Here's how the part is built. I have some questions about the finished solid (model axes, mm). A direction names the side the tool comes from. Give positions to 0.01 mm unless a question says otherwise; leave off trailing zeros. Write each loop counter-clockwise with the first axis right and the second up, starting at its lowest first coordinate (ties: lowest second). Pieces come first, ordered by that corner, then holes. Notation, with made-up numbers: M 55.5,25.5 L 77.5,25.5 A19 cw 77.5,56.5 Z; hole C 27,-11.75 d7. An arc over 180 degrees is marked long. Use one line per item in the form item = value. Start each with the question number.
from build123d import *

# Parameters (mm, degrees)
F1_DEPTH   = 228.6
F2_T       = -2.54
F4_W       = 223.52
F4_H       = 121.926114556
F5_DEPTH   = 134.112
F7_W       = 76.2
F7_H       = 177.8
F9_W       = 76.2
F9_H       = 177.8
F10_DEPTH  = 381
F8_FACE1_W = 76.2
F8_FACE1_H = 103.6678810409
F13_T      = -2.54
F11_W      = 533.4
F11_H      = 304.8
F11_W_2    = 76.2
F11_H_2    = 177.8
F14_DEPTH  = 5.08


# Not quite as in the source:
# - a shell that OpenCascade refuses in one call is made with other operations: the cavity is built on its own and cut out
# - a feature names something its author has since deleted; it is built from what else it names


with BuildPart() as f1:
    # F0 (on Right) → F1 (new body)
    with BuildSketch(Plane.YZ):
        Polygon((-381, 683.26), (0, 0), (145.4103401064, 0), (-235.5896598936, 683.26), align=None)
    extrude(amount=F1_DEPTH)

    # F2
    f2_openings = [f1.faces().sort_by_distance(p)[0] for p in [
        (114.3, -308.29483, 683.26),
    ]]
    offset(amount=F2_T, openings=f2_openings)

    # F4 (on face) → F5 (cut)
    with BuildSketch(Plane(origin=(0, 34.4790739886, -61.8450267372), x_dir=(1, 0, 0), z_dir=(0, -0.4869452699, 0.873432484))):
        with Locations((114.3, 63.503057278)):
            Rectangle(F4_W, F4_H)
    extrude(amount=F5_DEPTH, mode=Mode.SUBTRACT)

    # F7 (on offset) → F8 (join, up to the next surface of F1)
    with BuildSketch(Plane.XZ.offset(231.14)):
        with Locations((114.3, 139.7)):
            Rectangle(F7_W, F7_H)
    extrude(until=Until.NEXT, dir=(0, 1, 0))

    # F9 (on face) → F10 (join)
    with BuildSketch(Plane(origin=(0, 0, 50.8), x_dir=(1, 0, 0), z_dir=(0, 0, -1))):
        with Locations((114.3, 142.24)):
            Rectangle(F9_W, F9_H)
    extrude(amount=F10_DEPTH)

    # F8_face1 (on face) → F12 (join, up to the next surface of F1)
    with BuildSketch(Plane(origin=(114.3, -179.3060594796, 228.6), x_dir=(1, 0, 0), z_dir=(0, 0, 1))):
        Rectangle(F8_FACE1_W, F8_FACE1_H)
    extrude(until=Until.NEXT)

    # F13: a shell. OpenCascade refuses it in one call, so the cavity is built on its own and cut out:
    # the body offset inwards by the wall thickness, plus a prism from it out through each open face.
    f13_core = offset(f1.part, amount=F13_T, kind=Kind.INTERSECTION, mode=Mode.PRIVATE)
    f13_exits = [f13_core.faces().sort_by_distance(p)[0] for p in [
        (114.3, -55.88, -137.16),
    ]]
    add(f13_core, mode=Mode.SUBTRACT)
    extrude(f13_exits, amount=-F13_T, mode=Mode.SUBTRACT)

    # F11 (on face) → F14 (join)
    with BuildSketch(Plane(origin=(0, 0, -330.2), x_dir=(1, 0, 0), z_dir=(0, 0, -1))):
        with Locations((114.3, 104.14)):
            Rectangle(F11_W, F11_H)
        with Locations((114.3, 142.24)):
            Rectangle(F11_W_2, F11_H_2, mode=Mode.SUBTRACT)
        with Locations((114.3, 142.24)):
            Rectangle(F11_W_2, F11_H_2)
    extrude(amount=F14_DEPTH)


solid = f1.part
1) Will these pins go through, and if not, where does the flat tip stop? P1, Ø5, axis at x = 35.5, y = -270.5, coming from the -Z side; P2, Ø1.5, axis at x = 127.5, z = -332.5, coming from the -Y side; P3, Ø23, axis at x = 118.5, z = 146, coming from the -Y side.
2) Please list where these lines run through material, in increasing order: line 1 (X direction, y = -201.5, z = -76.5); line 2 (X direction, y = 88.5, z = 88); line 3 (Z direction, x = 217, y = -148).
3) On a 3-axis mill with a long thin cutter (end or side, diameter ignored), from which of +Z, -Z, +X, -X, +Y, -Y can I reach the whole of each face in a straight line? I mean faces 4 (the face through (226.06, -119, 369)), 5 (the face through (114, -41, 50.8)), 6 (the face through (114, 2, 0)), 7 (the face through (115, -142, -327.66)). Say none if no direction works.
4) Suppose I cut it at B-B, the plane z = -141.5. List the corners of the cut face in (x, y) for me, and give its area (3 significant figures).
5) Suppose I cut it at A-A, the plane x = 49. State how many separate pieces and enclosed holes the cut face has, and give its area (3 significant figures).
6) Thinking about a two-plate mould opening in Y: for faces 1 (the face through (0, -139, 343)), 2 (the face through (112.7, -42.423, 336.847)), 3 (the face through (2.54, -119, 369)), which applies, released by +Y, released by -Y, zero draft, split by the parting line, or undercut?
7) Suppose I cut it at D-D, the plane z = 102. List the corners of the cut face in (x, y) for me, and give its area (3 significant figures).
Checks:
q1.P1 = 480.61
q1.P2 = -256.54
q1.P3 = -231.14
q2.line_1 = 76.2 to 78.74, 149.86 to 152.4
q2.line_2 = 0 to 2.54, 226.06 to 228.6
q2.line_3 = -335.28 to -330.2, 265.41 to 270.63, 520.97 to 526.18
q3.face_4 = none
q3.face_5 = +X, -X
q3.face_6 = +X, -X, +Y
q3.face_7 = +Y
q4.outline = M 76.2,-231.14 L 152.4,-231.14 L 152.4,-53.34 L 149.86,-53.34 L 149.86,-228.6 L 78.74,-228.6 L 78.74,-53.34 L 76.2,-53.34 Z
q4.area = 1,080 mm^2
q5.separate_pieces = 3
q5.enclosed_holes = 0
q5.area = 5,520 mm^2
q6.face_1 = zero draft
q6.face_2 = released by +Y
q6.face_3 = undercut
q7.outline = M 0,-56.88 L 76.2,-56.88 L 76.2,-231.14 L 152.4,-231.14 L 152.4,-56.88 L 228.6,-56.88 L 228.6,88.53 L 0,88.53 Z; hole M 2.54,-53.97 L 226.06,-53.97 L 226.06,85.64 L 2.54,85.64 Z; hole M 78.74,-228.6 L 149.86,-228.6 L 149.86,-56.88 L 78.74,-56.88 Z
q7.area = 3,100 mm^2
